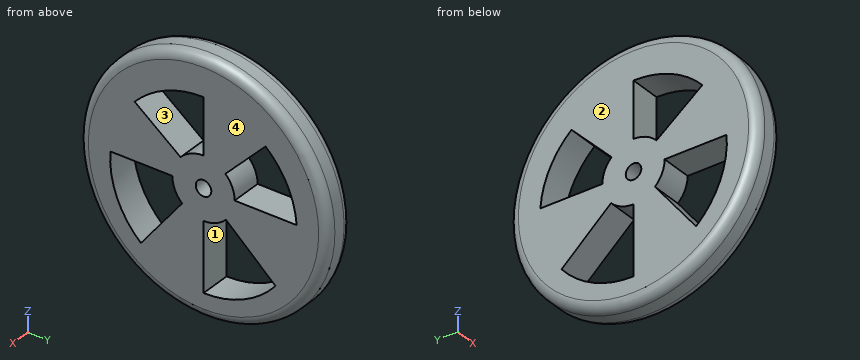
```python
from build123d import *

# Parameters (mm, degrees)
F0_R     = 101.6
F1_DEPTH = 25.4
F3_DEPTH = 25.4
F4_R     = 7.62
F5_R     = 6.35
F6_DEPTH = 25.4


with BuildPart() as f1:
    # F0 (on Right) → F1 (new body)
    with BuildSketch(Plane.YZ):
        Circle(F0_R)
    extrude(amount=F1_DEPTH)

    # F2 (on face) → F3 (cut)
    with BuildSketch(Plane.YZ.offset(25.4)):
        with BuildLine():
            Line((-51.087433, -61.850464), (-17.482547, -18.426083))
            ThreePointArc((-17.482547, -18.426083), (-23.336845, -10.027545), (-25.4, 0))
            Line((-25.4, 0), (-76.01457, 0))
            ThreePointArc((-76.01457, 0), (-70.67602, -33.796775), (-51.087433, -61.850464))
        make_face()
        with BuildLine():
            Line((58.748065, -53.842163), (18.349848, -17.562547))
            ThreePointArc((18.349848, -17.562547), (9.976755, -23.358603), (0, -25.4))
            Line((0, -25.4), (0, -81.512741))
            ThreePointArc((0, -81.512741), (32.469201, -74.248878), (58.748065, -53.842163))
        make_face()
        with BuildLine():
            ThreePointArc((17.89198, 18.028784), (23.447988, 9.764828), (25.4, 0))
            Line((25.4, 0), (76.01457, 0))
            ThreePointArc((76.01457, 0), (68.385887, 28.299913), (50.639288, 51.626723))
            Line((50.639288, 51.626723), (17.89198, 18.028784))
        make_face()
        with BuildLine():
            ThreePointArc((-18.739308, 17.146379), (-10.238212, 23.245193), (0, 25.4))
            Line((0, 25.4), (0, 70.887259))
            ThreePointArc((0, 70.887259), (-30.706062, 64.426615), (-56.205274, 46.14022))
            Line((-56.205274, 46.14022), (-18.739308, 17.146379))
        make_face()
    extrude(amount=-F3_DEPTH, mode=Mode.SUBTRACT)

    # F4
    f4_edges = [f1.edges().sort_by_distance(p)[0] for p in [
        (25.4, -101.6, 0),
        (0, -101.6, 0),
    ]]
    fillet(f4_edges, radius=F4_R)

    # F5 (on face) → F6 (cut)
    with BuildSketch(Plane.YZ.offset(25.4)):
        Circle(F5_R)
    extrude(amount=-F6_DEPTH, mode=Mode.SUBTRACT)


solid = f1.part
```
Part model, mm, in its own coordinate system. Face numbers are marked on the shaded views. A direction names the side the tool comes from. Round coordinates to 2 decimals unless told otherwise and drop trailing zeros. Write each loop counter-clockwise with the first axis right and the second up, starting at its lowest first coordinate (ties: lowest second). Pieces come first, ordered by that corner, then holes. Notation, with made-up numbers: (-39.75, 65.25) -> (6.25, 65.25) arc R15 ccw to (6.25, 81.25) -> close; hole circle Ø7 at (68.5, -33). An arc over 180 degrees is marked (long way). Return JSON: item names as keys, results as strings. Group by question number.
Q1. Which spindle directions (+Z, -Z, +X, -X, +Y, -Y) get a long thin tool onto all of the face, cutting with end or side? Do the marked faces 1 and 2. Say none if no direction does.
Q2. Pin check, flat tips, straight feed: pin 1 (4 mm diameter, centred on x = 6.5, z = 64, fed in from -Y); pin 2 (12.5 mm diameter, centred on x = 15.5, z = 41, fed in from -Y); pin 3 (1.5 mm diameter, centred on x = 7.5, z = 72, fed in from -Y). Stop position of each tip, or through.
Q3. Probe L1, parallel to Y at x = 1.5, z = -43; L2, parallel to Y at x = 5.75, z = 1; L3, parallel to Z at x = 13.25, y = 52. List the from-to ranges inside material, lowest first. Write a range as [from, to].
Q4. Saw through at A-A on x = 21.5. Write the cut outline in (y, z).
Q5. Saw through at B-B on y = -29. State how many separate pieces and enclosed holes the cut face has, plus the area to 3 significant figures.
Q6. Saw through at C-C on x = 4.5. Write the cut outline in (y, z).
Q7. Mould opens along Z. For the marked faces 3 and 4 say: pulls with the +Z half, pulls with the -Z half, needs draft (parallel to the pull), parting line crosses it, or undercut.
Answer:
{
 "1": {"face 1": "+X, -X", "face 2": "+Z, -Z, -X, +Y, -Y"},
 "2": {"pin 1": "y = -80.42", "pin 2": "y = -95.47", "pin 3": "y = -72.43"},
 "3": {"L1": "[-88.64, -66.23], [-36.5, 0], [46.68, 88.64]", "L2": "[-101.36, -6.27], [6.27, 25.38], [75.94, 101.36]", "L3": "[-87.28, -61.01], [-47.78, 0], [50.39, 87.28]"},
 "4": {"outline": "circle Ø201.26 at (0, 0); hole (-76.01, 0) arc R76.2 ccw to (-51.09, -61.85) -> (-17.48, -18.43) arc R25.4 cw to (-25.4, 0) -> close; hole (-56.21, 46.14) -> (-18.74, 17.15) arc R25.4 cw to (0, 25.4) -> (0, 70.89) arc R76.2 ccw to start; hole circle Ø12.7 at (0, 0); hole (0, -81.51) arc R76.2 ccw to (58.75, -53.84) -> (18.35, -17.56) arc R25.4 cw to (0, -25.4) -> close; hole (17.89, 18.03) arc R25.4 cw to (25.4, 0) -> (76.01, 0) arc R76.2 ccw to (50.64, 51.63) -> close"},
 "5": {"separate pieces": "3", "enclosed holes": "0", "area": "3,030 mm2"},
 "6": {"outline": "circle Ø201.86 at (0, 0); hole (-76.01, 0) arc R76.2 ccw to (-51.09, -61.85) -> (-17.48, -18.43) arc R25.4 cw to (-25.4, 0) -> close; hole (-56.21, 46.14) -> (-18.74, 17.15) arc R25.4 cw to (0, 25.4) -> (0, 70.89) arc R76.2 ccw to start; hole circle Ø12.7 at (0, 0); hole (0, -81.51) arc R76.2 ccw to (58.75, -53.84) -> (18.35, -17.56) arc R25.4 cw to (0, -25.4) -> close; hole (17.89, 18.03) arc R25.4 cw to (25.4, 0) -> (76.01, 0) arc R76.2 ccw to (50.64, 51.63) -> close"},
 "7": {"face 3": "undercut", "face 4": "needs draft"}
}
